Build history of the part. All positions in model axes, mm. A direction names the side the tool comes from. Give positions to 0.01 mm unless a question says otherwise; leave off trailing zeros. Loops run counter-clockwise (first coordinate to the right, second up) from the corner with the lowest first, then second, coordinate; pieces in that order, holes last. Notation, with made-up numbers: (25.25, -38.75) -> (65.25, -38.75) arc R24 cw to (65.25, -6.75) -> close; hole circle Ø3 at (35, 39). An arc over 180 degrees is marked (long way). One line per question, with ' | ' between items. Start each with the question number.
(1) Slice it at A-A, the plane x = -43. Write the cut outline in (y, z), then the cut area to 3 significant figures.
(2) 3-axis set-ups, long thin cutter, end or side, ignore diameter. For faces 4 (the face through (-20, -31, 23)), 5 (the face through (-4, 0, 43)), 6 (the face through (-14, 28, 43)), 7 (the face through (-32, -1, 0)): which of +Z, -Z, +X, -X, +Y, -Y reach the whole face in a straight line?
(3) Slice it at B-B, the plane z = 28. Write the cut outline in (x, y), then the cut area to 3 significant figures.
(4) Mould opens along Z. For faces 1 (the face through (-14, -28, 3)), 2 (the face through (-32, -1, 46)), 3 (the face through (-1.5, 0.07, 44.48)) say: pulls with the +Z half, pulls with the -Z half, needs draft (parallel to the pull), parting line crosses it, or undercut.
(5) Slice it at D-D, the plane y = -10. Write the cut outline in (x, z), then the cut area to 3 significant figures.
(6) Drill centre lines: L1, parallel to Y at x = -43, z = 45.4; L2, parallel to X at y = 20, z = 1.45; L3, parallel to Z at x = -14.5, y = -7.5. Where is each one in solid material? Low to high. Write a range as from..to.
(7) Slice it at C-C, the plane x = 4. Write the cut outline in (y, z).
(8) Flat gauge pins, fed straight in: pin 1 Ø12 at (x, z) = (2, 24) entering from +Y; pin 2 Ø4 at (y, z) = (1, 40) entering from +X. Where does each tip first touch, or does it go through?
```python
from build123d import *

# Parameters (mm, degrees)
BOSS_EXTRU_1_DEPTH           = 3
ESQUISSE2_W                  = 3
ESQUISSE2_H                  = 40
BOSS_EXTRU_2_DEPTH           = 20
ENL_V_MAT_EXTRU_1_DEPTH      = 90.844309781
ENL_V_MAT_EXTRU_1_DEPTH_BACK = 90.844309781
ESQUISSE3_R                  = 1.5


with BuildPart() as part:
    # Esquisse1 → Boss.-Extru.1 (new body)
    with BuildSketch(Plane.XY):
        Polygon((-66, 40), (-20, 40), (0, 23), (20, 23), (20, 0), (0, 0), (-66, 0), align=None)
    extrude(amount=BOSS_EXTRU_1_DEPTH)

    # Esquisse2 → Boss.-Extru.2 (add)
    with BuildSketch(Plane.XY.offset(3)):
        Polygon((20, 23), (-20, 23), (-20, 40), (-23, 40), (-23, 0), (-20, 0), (-20, 20), (20, 20), align=None)
        with Locations((-64.5, 20)):
            Rectangle(ESQUISSE2_W, ESQUISSE2_H)
    extrude(amount=BOSS_EXTRU_2_DEPTH)

    # Symétrie1: part across plane


with BuildPart() as part_1:
    add(part.part)
    add(part.part.mirror(Plane(origin=(20, 0, 3), x_dir=(0, 0, 1), z_dir=(0, 1, 0))))

    # Symétrie2: part across plane


with BuildPart() as part_2:
    add(part_1.part)
    add(part_1.part.mirror(Plane.XY.offset(23)))

    # Esquisse3 → Enlèv. mat.-Extru.1 (cut, two sides: drawn at the far end of the back side and taken through both)
    with BuildSketch(Plane.XY.offset(46).offset(-ENL_V_MAT_EXTRU_1_DEPTH_BACK)):
        with Locations((-43, 20)):
            Circle(ESQUISSE3_R)
        with Locations((-43, -20)):
            Circle(ESQUISSE3_R)
        Circle(ESQUISSE3_R)
    extrude(amount=ENL_V_MAT_EXTRU_1_DEPTH + ENL_V_MAT_EXTRU_1_DEPTH_BACK, mode=Mode.SUBTRACT)


solid = part_2.part
```
Final values:
1) outline: (-40, 0) -> (-21.5, 0) -> (-21.5, 3) -> (-40, 3) -> close; (-40, 43) -> (-21.5, 43) -> (-21.5, 46) -> (-40, 46) -> close; (-18.5, 0) -> (18.5, 0) -> (18.5, 3) -> (-18.5, 3) -> close; (-18.5, 43) -> (18.5, 43) -> (18.5, 46) -> (-18.5, 46) -> close; (21.5, 0) -> (40, 0) -> (40, 3) -> (21.5, 3) -> close; (21.5, 43) -> (40, 43) -> (40, 46) -> (21.5, 46) -> close | area: 444 mm2
2) face 4: +X, -Y | face 5: +X | face 6: +X, +Y | face 7: -Z, +X, -X, +Y, -Y
3) outline: (-66, -40) -> (-63, -40) -> (-63, 40) -> (-66, 40) -> close; (-23, -40) -> (-20, -40) -> (-20, -23) -> (20, -23) -> (20, -20) -> (-20, -20) -> (-20, 20) -> (20, 20) -> (20, 23) -> (-20, 23) -> (-20, 40) -> (-23, 40) -> close | area: 720 mm2
4) face 1: undercut | face 2: pulls with the +Z half | face 3: needs draft
5) outline: (-66, 0) -> (20, 0) -> (20, 3) -> (-20, 3) -> (-20, 43) -> (20, 43) -> (20, 46) -> (-66, 46) -> close; hole (-63, 3) -> (-23, 3) -> (-23, 43) -> (-63, 43) -> close | area: 756 mm2
6) L1: -40..-21.5, -18.5..18.5, 21.5..40 | L2: -66..-44.5, -41.5..20 | L3: 0..3, 43..46
7) outline: (-23, 0) -> (23, 0) -> (23, 46) -> (-23, 46) -> close; hole (-20, 3) -> (20, 3) -> (20, 43) -> (-20, 43) -> close
8) pin 1: y = 23 | pin 2: x = -20
